```python
from build123d import *

# Parameters (mm, degrees)
SKETCH4_R               = 4
SKETCH4_R_2             = 2.5
SKETCH4_R_3             = 1.75
BOSS_EXTRUDE2_DEPTH     = 2
FILLET3_R               = 1
CUT_EXTRUDE1_DEPTH      = 225.288694563
CUT_EXTRUDE1_DEPTH_BACK = 225.288694563
SKETCH6_R               = 0.767868533
SKETCH6_R_2             = 0.771761199
SKETCH6_R_3             = 0.768034618
SKETCH6_R_4             = 0.795284138


with BuildPart() as part:
    # Sketch4 → Boss-Extrude2 (new, symmetric)
    with BuildSketch(Plane.XY):
        with BuildLine():
            ThreePointArc((-37.367897149, 54.387204077), (-49.125443785, 128.867751214), (-54.236117249, 204.097218987))
            ThreePointArc((-54.236117249, 204.097218987), (-41.377914553, 217.590696941), (-27.867941637, 204.749826423))
            ThreePointArc((-27.867941637, 204.749826423), (-20.824641361, 133.142032668), (-3.576140657, 63.286657579))
            ThreePointArc((-3.576140657, 63.286657579), (-15.763142173, 40.957044634), (-37.367897149, 54.387204077))
        make_face()
        with Locations((-20.22, 57.88)):
            Circle(SKETCH4_R, mode=Mode.SUBTRACT)
        with Locations((-41.051610566, 204.406598272)):
            Circle(SKETCH4_R_2, mode=Mode.SUBTRACT)
        with Locations((-37.268473007, 154.549924996)):
            Circle(SKETCH4_R_3, mode=Mode.SUBTRACT)
        with Locations((-30.482103359, 106.815562065)):
            Circle(SKETCH4_R_3, mode=Mode.SUBTRACT)
    extrude(amount=BOSS_EXTRUDE2_DEPTH, both=True)

    # Fillet3
    fillet3_edges = [part.edges().sort_by_distance(p)[0] for p in [
        (-41.377914553, 217.590696941, -2),
        (-20.824641361, 133.142032668, -2),
        (-15.763142173, 40.957044634, -2),
        (-49.125443785, 128.867751214, -2),
        (-49.125443785, 128.867751214, 2),
        (-15.763142173, 40.957044634, 2),
        (-20.824641361, 133.142032668, 2),
        (-41.377914553, 217.590696941, 2),
    ]]
    fillet(fillet3_edges, radius=FILLET3_R)

    # Sketch6 → Cut-Extrude1 (cut, two sides: drawn at the far end of the back side and taken through both)
    with BuildSketch(Plane(origin=(0, 0, -2), x_dir=(-1, 0, 0), z_dir=(0, 0, -1)).offset(-CUT_EXTRUDE1_DEPTH_BACK)):
        with Locations((24.81448084, 64.15193249)):
            Circle(SKETCH6_R)
        with Locations((26.515189166, 53.299256498)):
            Circle(SKETCH6_R_2)
        with Locations((15.627794635, 51.635896996)):
            Circle(SKETCH6_R_3)
        with Locations((13.984842021, 62.426172158)):
            Circle(SKETCH6_R_4)
    extrude(amount=CUT_EXTRUDE1_DEPTH + CUT_EXTRUDE1_DEPTH_BACK, mode=Mode.SUBTRACT)


solid = part.part
```
Verification items for the finished model (mm, model axes). Coordinates: 2 decimals unless noted, no trailing zeros. Put each result on its own line as item: value.
1. Thickness scan on line 1 (Y direction, x = -31.5, z = 1.8); line 2 (X direction, y = 57.5, z = 0.4); line 3 (X direction, y = 56, z = -0.75). Record the ranges inside material, lowest first.
Result set:
line 1: y = 45.03 to 105.39, 108.24 to 212.91
line 2: x = -38 to -24.2, -16.24 to -2.72
line 3: x = -37.69 to -23.75, -16.69 to -2.82
2. Section check A-A, the plane z = 0.2. Give the number of separate pieces and of enclosed holes in the cut face, then the cut area to 3 significant figures.
Result set:
separate pieces: 1
enclosed holes: 8
area: 5,010 mm^2
3. Gauge pin test, flat ends, axial feed: P1, Ø2, axis at x = -45.5, z = -1, coming from the +Y side; P2, Ø1.5, axis at y = 86, z = -1, coming from the +X side. Record the tip position at first contact, or that the pin passes through.
Result set:
P1: stops at y = 217.14
P2: stops at x = -10.16
4. Mould release check, pull along Y, two halves, no side actions. Record for faces 1 (the face through (-36.328, 156.026, -0.028)), 2 (the face through (-34, 130, 2)), 3 (the face through (-49.007, 127.818, 0.014)), 4 (the face through (-30.861, 105.107, -0.028)): pulls with the +Y half, pulls with the -Y half, needs draft (parallel to the pull), parting line crosses it, or undercut.
Result set:
face 1: undercut
face 2: needs draft
face 3: pulls with the -Y half
face 4: undercut
